from build123d import *

# Parameters (mm, degrees)
F0_W     = 254
F0_H     = 9.267491
F1_DEPTH = 2.54
F2_R     = 2.54
F6_DEPTH = 2.54


with BuildPart() as f1:
    # F0 (on Front) → F1 (new body)
    with BuildSketch(Plane.XZ):
        with Locations((-2.819128, 33.181484)):
            Rectangle(F0_W, F0_H)
    extrude(amount=F1_DEPTH)

    # F2
    f2_edges = [f1.edges().sort_by_distance(p)[0] for p in [
        (124.180872, -1.27, 37.81523),
        (124.180872, -1.27, 28.547739),
        (-129.819128, -1.27, 37.81523),
        (-129.819128, -1.27, 28.547739),
    ]]
    fillet(f2_edges, radius=F2_R)

    # F3 (on face) + F4 (on face) + F5 (on face) → F6 (join)
    with BuildSketch(Plane.XZ.offset(2.54)):
        Polygon((-77.991536, 28.547739), (-74.369276, 28.547739), (-71.807952, 31.109063), (-71.807952, 34.731323), (-74.369276, 37.292647), (-77.991536, 37.292647), (-80.55286, 34.731323), (-80.55286, 31.109063), align=None)
    with BuildSketch(Plane.XZ.offset(2.54)):
        Polygon((5.658443, 28.784776), (9.283109, 28.784776), (11.846135, 31.347802), (11.846135, 34.972468), (9.283109, 37.535494), (5.658443, 37.535494), (3.095417, 34.972468), (3.095417, 31.347802), align=None)
    with BuildSketch(Plane.XZ.offset(2.54)):
        Polygon((74.223366, 28.135227), (78.068468, 28.135227), (78.48098, 28.547739), (73.810854, 28.547739), align=None)
        Polygon((73.810854, 28.547739), (78.48098, 28.547739), (80.787366, 30.854125), (80.787366, 34.699227), (78.068468, 37.418125), (74.223366, 37.418125), (71.504468, 34.699227), (71.504468, 30.854125), align=None)
    extrude(amount=F6_DEPTH)


solid = f1.part
Check sheet for the modelled part. Datum: model origin and axes. Units: mm. Give positions to 0.01 mm unless a question says otherwise; leave off trailing zeros. Loops run counter-clockwise (first coordinate to the right, second up) from the corner with the lowest first, then second, coordinate; pieces in that order, holes last. Notation, with made-up numbers: M -38,75.5 L -25,75.5 A14 cw -25,81.5 Z; hole C -30,62 d3. An arc over 180 degrees is marked long. Answer as a JSON object with one key per item and string values. Group by question number.
Q1. Go/stop test with flat-tipped pins: P1, Ø1.3, axis at x = -14, y = -1, coming from the -Z side; P2, Ø1.3, axis at y = -3.5, z = 32.5, coming from the +X side; P3, Ø0.8, axis at x = 7, y = -3.5, coming from the +Z side. Record where each tip stops, or that it passes through.
Q2. Release check for a two-part mould opening along X. For faces 1 (the flat face through (-5, -2.54, 33)), 2 (the flat face through (76, -5.08, 33)) record: released by +X, released by -X, zero draft, split by the parting line, or undercut.
Q3. Cross-section at A-A on y = -3.7. Record the cut outline in (x, z), then the cut area to 3 significant figures.
Q4. Material ranges on line 1 along X through (y, z) = (-2.6, 34.25); line 2 along X through (y, z) = (-4.45, 31.25); line 3 along Y through (x, z) = (-67, 35.75), recorded low to high. Write a range as [from, to].
Q5. Cross-section at B-B on x = 26. Record the cut outline in (y, z), then the cut area to 3 significant figures.
Evaluation:
{
 "1": {"P1": "stops at z = 28.55", "P2": "stops at x = 80.79", "P3": "stops at z = 37.54"},
 "2": {"face 1": "undercut", "face 2": "zero draft"},
 "3": {"outline": "M -80.55,31.11 L -77.99,28.55 L -74.37,28.55 L -71.81,31.11 L -71.81,34.73 L -74.37,37.29 L -77.99,37.29 L -80.55,34.73 Z; M 3.1,31.35 L 5.66,28.78 L 9.28,28.78 L 11.85,31.35 L 11.85,34.97 L 9.28,37.54 L 5.66,37.54 L 3.1,34.97 Z; M 71.5,30.85 L 74.22,28.14 L 78.07,28.14 L 80.79,30.85 L 80.79,34.7 L 78.07,37.42 L 74.22,37.42 L 71.5,34.7 Z", "area": "198 mm2"},
 "4": {"line 1": "x = [-80.55, -71.81], [3.1, 11.85], [71.5, 80.79]", "line 2": "x = [-80.55, -71.81], [3.19, 11.75], [71.5, 80.79]", "line 3": "y = [-2.54, 0]"},
 "5": {"outline": "M -2.54,28.55 L 0,28.55 L 0,37.82 L -2.54,37.82 Z", "area": "23.5 mm2"}
}
